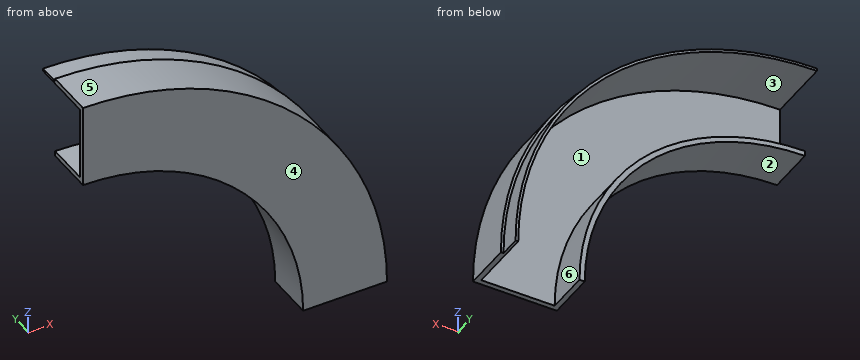
Autodesk Inventor part; units mm, degrees
ref_plane "YZ Plane" through (0, 0, 0) normal (1, 0, 0) x (0, 1, 0)
ref_plane "XZ Plane" through (0, 0, 0) normal (0, 1, 0) x (-1, 0, 0)
ref_plane "XY Plane" through (0, 0, 0) normal (0, 0, 1) x (1, 0, 0)
sketch "Sketch1" plane through (0, 0, 0) normal (1, 0, 0) x (0, 1, 0)
  line L0 (0, 0) -> (50.8, 0)
  line L1 (0, 133.35) -> (0, 184.15)
  line L2 (0, 184.15) -> (29.2989, 184.15)
  line L3 (73.025, 184.15) -> (73.025, 133.35)
  line L4 (3.175, 180.975) -> (3.175, 136.525)
  line L5 (69.85, 136.525) -> (69.85, 180.975)
  line L6 (29.2989, 148.3694) -> (29.2989, 120.4477)
  line L7 (41.9989, 148.9666) -> (41.9989, 122.6874)
  line L8 (0, 133.35) -> (29.2989, 133.35)
  line L9 (41.9989, 133.35) -> (73.025, 133.35)
  line L10 (3.175, 136.525) -> (29.2989, 136.525)
  line L11 (41.9989, 136.525) -> (69.85, 136.525)
  line L12 (35.6489, 182.5625) -> (41.9989, 182.5625)
  line L13 (41.9989, 182.5625) -> (41.9989, 180.975)
  line L14 (35.6489, 182.5625) -> (29.2989, 182.5625)
  line L15 (29.2989, 182.5625) -> (29.2989, 184.15)
  line L16 (69.85, 180.975) -> (41.9989, 180.975)
  line L17 (35.6489, 180.975) -> (3.175, 180.975)
  line L18 (35.6489, 170.617) -> (35.6489, 180.975)
  line L19 (35.6489, 184.15) -> (35.6489, 201.7381)
  line L20 (35.6489, 180.975) -> (41.9989, 180.975)
  point P0 (3.175, 180.975)
  point P1 (69.85, 136.525)
  dimension "d0" = 50.8
  dimension "d3" = 50.8
  dimension "d4" = 73.025
  dimension "d5" = 3.175
  dimension "d6" = 3.175
  dimension "d7" = 3.175
  dimension "d8" = 3.175
  dimension "d9" = 3.175
  dimension "d11" = 3.175
  dimension "d13" = 26.1239
  dimension "d14" = 12.7
  dimension "d16" = 133.35
  dimension "d17" = 3.175
  dimension "d18" = 3.175
  dimension "d19" = 6.35
  dimension "d21" = 6.35
  dimension "d22" = 6.35
revolve "Revolution1" add sketch "Sketch1" angle 180 about axis through (0, 0, 0) along (0, 1, 0)
sketch "Sketch2" plane through (0, 0, 133.35) normal (0, -1, 0) x (1, 0, 0)
  line L0 (0, -133.35) -> (197.7454, -133.35)
  line L1 (197.7454, -133.35) -> (197.7454, -342.2428)
  line L2 (197.7454, -342.2428) -> (0, -342.2428)
  line L3 (0, -342.2428) -> (0, -133.35)
extrude "Extrusion1" cut sketch "Sketch2" against normal through all
properties part number "Outer_Shell_Bottom_Quarter"
CAD build for the part. Positions are in the model's coordinates, mm. Face numbers are marked on the shaded views. A direction names the side the tool comes from. Round coordinates to 2 decimals unless told otherwise and drop trailing zeros. Order: outer loops, then holes, each group sorted by start corner. A loop starts at its lowest first (then second) coordinate and runs counter-clockwise, first axis right, second up. Notation, with made-up numbers: (-15.75, 0) -> (-9.75, 0) arc R12 ccw to (-9.75, 17) -> close; hole circle Ø11 at (-13, -24.75). An arc over 180 degrees is marked (long way). Write item = value, one per line.
(1) Cut at C-C (x = 16.5). Write the cut outline in (y, z) (3 decimals).
Answers follow:
outline = (0, 132.325) -> (29.299, 132.325) -> (29.299, 135.524) -> (3.175, 135.524) -> (3.175, 180.221) -> (41.999, 180.221) -> (41.999, 181.815) -> (29.299, 181.815) -> (29.299, 183.409) -> (0, 183.409) -> close
(2) Drill centre lines: L1, parallel to Y at x = 161, z = 8.5 (3 decimals); L2, parallel to Z at x = 55.5, y = 4; L3, parallel to X at y = 18, z = 74. Where is each one in solid material? Low to high.
Answers follow:
L1 = 0 to 3.175
L2 = 121.25 to 124.74, 172.25 to 175.59
L3 = 110.93 to 114.73, 165.15 to 168.63
(3) 3-axis set-ups, long thin cutter, end or side, ignore diameter. For the marked faces 5 and 6: which of +Z, -Z, +X, -X, +Y, -Y reach the whole face in a straight line?
Answers follow:
face_5 = +Z, +X, +Y, -Y
face_6 = +Y
(4) Pull direction X, two halves, no side cores. Call the marked faces 1, 2, 3 and 4: +X half, -X half, draft (parallel to the pull), parting line (faces both ways), or undercut.
Answers follow:
face_1 = undercut
face_2 = -X half
face_3 = undercut
face_4 = draft
(5) Cut at A-A (y = 18). Write the cut outline in (x, z) (3 decimals), plus the area to 3 significant figures.
Answers follow:
outline = (0, 133.35) arc R133.35 cw to (133.35, 0) -> (136.525, 0) arc R136.525 ccw to (0, 136.525) -> close; (0, 180.975) arc R180.975 cw to (180.975, 0) -> (184.15, 0) arc R184.15 ccw to (0, 184.15) -> close
area = 1,580 mm²
(6) Cut at B-B (z = 117.5). Write the cut outline in (x, y) (3 decimals).
Answers follow:
outline = (63.055, 0) -> (141.792, 0) -> (141.792, 29.299) -> (139.724, 29.299) -> (139.724, 41.999) -> (137.643, 41.999) -> (137.643, 3.175) -> (69.519, 3.175) -> (69.519, 29.299) -> (63.055, 29.299) -> close
(7) Flat gauge pins, fed straight in: P1, Ø2, axis at x = 140.5, y = 14, coming from the +Z side; P2, Ø5, axis at x = 78.5, y = 18, coming from the -Z side; P3, Ø6, axis at x = 34.5, y = 20.5, coming from the +Z side. Where does each tip first touch, or does it go through?
Answers follow:
P1 = 120.21
P2 = 105.93
P3 = 181.44
